Answer from the drawing. Dimensions are ordinates in mm from the lowest x, y and z of the part. A direction names the side the tool comes from. Coordinates: 2 decimals unless noted, no trailing zeros. Order: outer loops, then holes, each group sorted by start corner. A loop starts at its lowest first (then second) coordinate and runs counter-clockwise, first axis right, second up. Notation, with made-up numbers: (0, -20) - (58, -20) arc R9 cw to (58, -13) - close; hole circle Ø4 at (39, 70.25). An arc over 180 degrees is marked (long way). Answer as a JSON object with one key per item and string values. Group by question number.
1) Each of these flat-tipped pins is pushed along its axis until it touches: P1, Ø1, axis at x = 116.5, z = 17, coming from the +Y side (3 decimals); P2, Ø4, axis at x = 69, y = 13.5, coming from the +Z side (3 decimals); P3, Ø3, axis at x = 17, y = 34, coming from the -Z side. Where does it stop, or does it pass through?
2) Section B-B (z = 19.05) is taken. Give the vertices of the cut face in (x, y) (1 decimal).
3) Section C-C (y = 19.5) is taken. Give the vertices of the cut face in (x, z) (3 decimals).
4) Find the intervals of material crossed by line 1 along Y through (x, z) = (237, 1); line 2 along Z through (x, y) = (161, 28) (3 decimals), in increasing order.
5) A tool of negligible diameter and unlimited length cuts with its end or side. For the marked faces 1 and 2, from which of +Z, -Z, +X, -X, +Y, -Y can it reach the whole face along a straight path? Write none if from no direction.
6) Section D-D (x = 88) is taken. Give the vertices of the cut face in (y, z) (3 decimals).
7) Section A-A (x = 25.4) is taken. Give the vertices of the cut face in (y, z) (1 decimal).
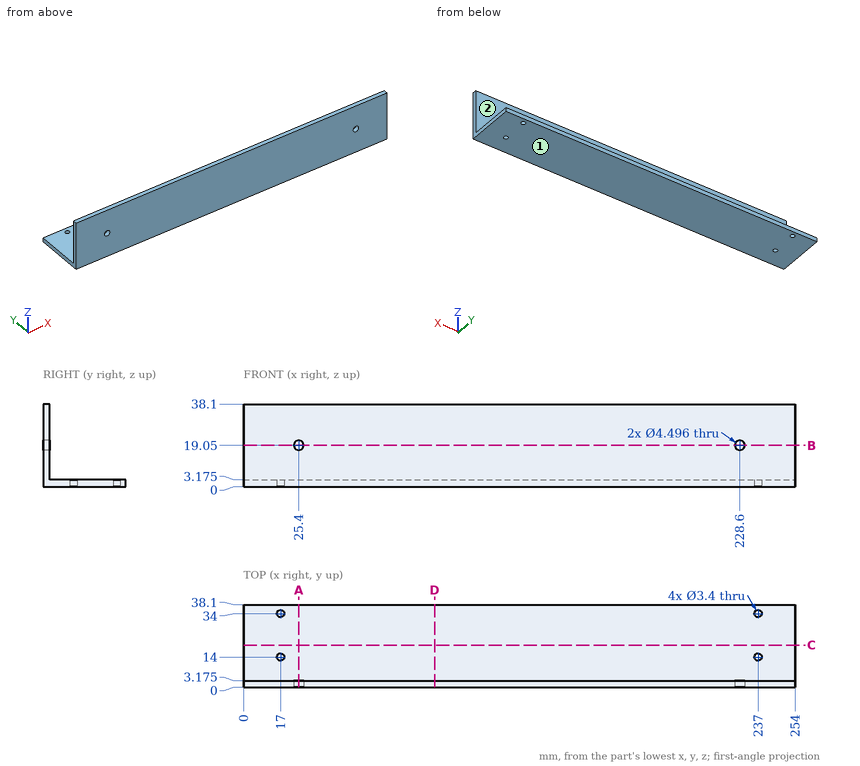
Report:
{
 "1": {"P1": "stops at y = 3.175", "P2": "stops at z = 3.175", "P3": "passes through"},
 "2": {"outline": "(0, 0) - (23.2, 0) - (23.2, 3.2) - (0, 3.2) - close; (27.6, 0) - (226.4, 0) - (226.4, 3.2) - (27.6, 3.2) - close; (230.8, 0) - (254, 0) - (254, 3.2) - (230.8, 3.2) - close"},
 "3": {"outline": "(0, 0) - (254, 0) - (254, 3.175) - (0, 3.175) - close"},
 "4": {"line 1": "y = 0 to 12.3, 15.7 to 32.3, 35.7 to 38.1", "line 2": "z = 0 to 3.175"},
 "5": {"face 1": "-Z, +X, -X, +Y, -Y", "face 2": "+Z, +X, -X, +Y"},
 "6": {"outline": "(0, 0) - (38.1, 0) - (38.1, 3.175) - (3.175, 3.175) - (3.175, 38.1) - (0, 38.1) - close"},
 "7": {"outline": "(0, 0) - (38.1, 0) - (38.1, 3.2) - (3.2, 3.2) - (3.2, 16.8) - (0, 16.8) - close; (0, 21.3) - (3.2, 21.3) - (3.2, 38.1) - (0, 38.1) - close"}
}
